The model under review builds one solid part; all positions refer to its coordinate system, in mm. A direction names the side the tool comes from. Coordinates: 2 decimals unless noted, no trailing zeros. Write each loop counter-clockwise with the first axis right and the second up, starting at its lowest first coordinate (ties: lowest second). Pieces come first, ordered by that corner, then holes.
```python
from build123d import *

# Parameters (mm, degrees)
F2_ANGLE       = 180
F1_R           = 70.7106781187
F3_DEPTH       = 3
F5_ANGLE       = 180
F8_W           = 100
F8_H           = 100
F9_DEPTH       = 25
F11_W          = 100
F11_H          = 100
F12_DEPTH      = 25
F13_R          = 35
F14_DEPTH      = 26.501
F14_DEPTH_BACK = 23.501


with BuildPart() as f2:
    # F1 (on Top) → F2 (revolve)
    with BuildSketch(Plane.XY):
        with BuildLine():
            ThreePointArc((-46.5, 0), (0, -46.5), (46.5, 0))
            Line((46.5, 0), (-46.5, 0))
        make_face()
    revolve(axis=Axis((0, 0, 0), (1, 0, 0)), revolution_arc=F2_ANGLE)

    # F1 (on Top) → F3 (join)
    with BuildSketch(Plane.XY):
        Circle(F1_R)
        with BuildLine():
            ThreePointArc((-46.5, 0), (0, 46.5), (46.5, 0))
            ThreePointArc((46.5, 0), (0, -46.5), (-46.5, 0))
        make_face(mode=Mode.SUBTRACT)
        with BuildLine():
            Line((-46.5, 0), (46.5, 0))
            ThreePointArc((46.5, 0), (0, 46.5), (-46.5, 0))
        make_face()
        with BuildLine():
            ThreePointArc((-46.5, 0), (0, -46.5), (46.5, 0))
            Line((46.5, 0), (-46.5, 0))
        make_face()
    extrude(amount=F3_DEPTH)

    # F4 (on face) → F5 (revolve)
    with BuildSketch(Plane.XY.offset(3)):
        with BuildLine():
            Line((46.5, 0), (-46.5, 0))
            ThreePointArc((-46.5, 0), (0, -46.5), (46.5, 0))
        make_face()
    revolve(axis=Axis((0, 0, 3), (-1, 0, 0)), revolution_arc=F5_ANGLE)

    # F8 (on plane+point) → F9 (cut)
    with BuildSketch(Plane.XY.offset(26.5)):
        Rectangle(F8_W, F8_H)
    extrude(amount=F9_DEPTH, mode=Mode.SUBTRACT)

    # F11 (on plane+point) → F12 (cut)
    with BuildSketch(Plane.XY.offset(-23.5)):
        Rectangle(F11_W, F11_H)
    extrude(amount=-F12_DEPTH, mode=Mode.SUBTRACT)

    # F13 (on Top) → F14 (cut, two sides)
    with BuildSketch(Plane.XY) as f14_sk:
        Circle(F13_R)
    extrude(amount=F14_DEPTH, mode=Mode.SUBTRACT)
    extrude(f14_sk.sketch, amount=-F14_DEPTH_BACK, mode=Mode.SUBTRACT)


solid = f2.part
```
Item 1: Take a section at A-A, the plane x = 0. Write out the cut boundary in (y, z), plus the area to 3 significant figures.
Solved:
outline: (-70.71, 0) - (-46.5, 0) arc R46.5 ccw to (-40.12, -23.5) - (-35, -23.5) - (-35, 26.5) - (-40.12, 26.5) arc R46.5 ccw to (-46.5, 3) - (-70.71, 3) - close; (35, -23.5) - (40.12, -23.5) arc R46.5 ccw to (46.5, 0) - (70.71, 0) - (70.71, 3) - (46.5, 3) arc R46.5 ccw to (40.12, 26.5) - (35, 26.5) - close
area: 1,100 mm2
Item 2: To check wall thickness, follow line 1 along Y through (x, z) = (0.5, -1); line 2 along Z through (x, y) = (43, -50.5); line 3 along Y through (x, z) = (3, 10). State the ranges of each line that lie inside material, in increasing order.
Solved:
line 1: y = -46.49 to -35, 35 to 46.49
line 2: z = 0 to 3
line 3: y = -45.87 to -34.87, 34.87 to 45.87
Item 3: Machinability: for faces 4 (the face through (46, -15, 3)), 5 (the face through (3, 36, 26.5)), 6 (the face through (46, -15, 0)), which of the approach directions +Z, -Z, +X, -X, +Y, -Y give a long, thin tool a straight path to every point of the face, cutting with its end or side? Answer none if there is none.
Solved:
face 4: +Z
face 5: +Z, +X, -X, +Y, -Y
face 6: -Z
Item 4: For pin 1 (3 mm diameter, centred on x = 42.5, y = 46, fed in from +Z); pin 2 (1.5 mm diameter, centred on x = 18, y = 37.5, fed in from +Z); pin 3 (4 mm diameter, centred on y = -18, z = -6, fed in from +X), all flat-tipped, find the tip position at first contact; note any pin that passes through.
Solved:
pin 1: stops at z = 3
pin 2: stops at z = 25.22
pin 3: stops at x = 43.29
Item 5: Take a section at C-C, the plane z = 6.5. Write out the cut boundary in (x, y), plus the area to 3 significant figures.
Solved:
outline: circle Ø92.74 at (0, 0); hole circle Ø70 at (0, 0)
area: 2,910 mm2
Item 6: Take a section at D-D, the plane y = 50. Write out the cut boundary in (x, z).
Solved:
outline: (-50, 0) - (50, 0) - (50, 3) - (-50, 3) - close
Item 7: Mouldability with a two-part tool opening along X and no side actions: class faces 1 (the face through (67.445, 21.24, 1.479)), 2 (the face through (-28, -21, 2)), 3 (the face through (3, 36, -23.5)) as pulls with the +X half, pulls with the -X half, needs draft (parallel to the pull), parting line crosses it, or undercut.
Solved:
face 1: parting line crosses it
face 2: undercut
face 3: needs draft
